Check sheet for the drawn part. Datum: minimum x, y, z corner. Units: mm. Coordinates: 2 decimals unless noted, no trailing zeros. Write each loop counter-clockwise with the first axis right and the second up, starting at its lowest first coordinate (ties: lowest second). Pieces come first, ordered by that corner, then holes. Notation, with made-up numbers: M -26,5.25 L -22,5.25 A25 ccw -22,33.25 Z; hole C 32.25,78.5 d4. An arc over 180 degrees is marked long. Answer as CSV lines item,"result". Start each with the question number.
Q1. Mould release check, pull along Y, two halves, no side actions. Record for the marked faces 1 and 2: pulls with the +Y half, pulls with the -Y half, needs draft (parallel to the pull), parting line crosses it, or undercut.
Q2. Sectioned sample at A-A, the plane x = 49. Record the cut outline in (y, z).
Q3. Sectioned sample at B-B, the plane y = 19. Record the cut outline in (x, z).
Q4. Thickness scan on line 1 along X through (y, z) = (7, 2.8); line 2 along Y through (x, z) = (71.5, 2.65); line 3 along Z through (x, y) = (41, 17). Record the ranges inside material, lowest first. Write a range as from..to.
Q5. Depth check by flat-ended pin: pin 1 Ø0.5 at (x, z) = (81.5, 3.5) entering from -Y; pin 2 Ø5.5 at (x, y) = (44, 9) entering from +Z; pin 3 Ø1.5 at (y, z) = (15.5, 2.5) entering from -X. Enter the tip coordinate at first touch or a pass-through.
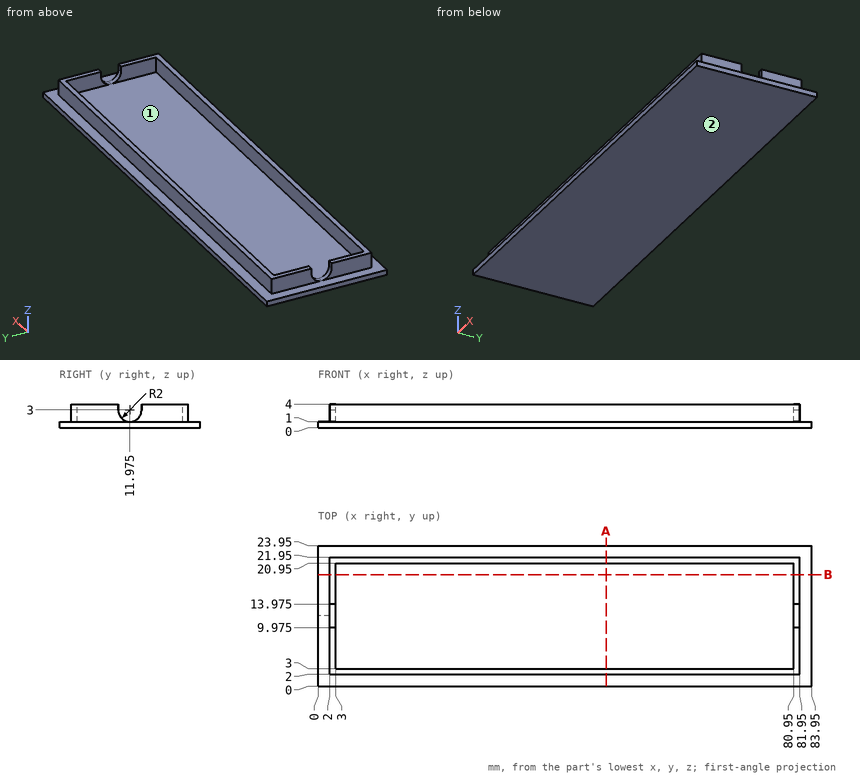
Output:
1,face 1,"undercut"
1,face 2,"needs draft"
2,outline,"M 0,0 L 23.95,0 L 23.95,1 L 21.95,1 L 21.95,4 L 20.95,4 L 20.95,1 L 3,1 L 3,4 L 2,4 L 2,1 L 0,1 Z"
3,outline,"M 0,0 L 83.95,0 L 83.95,1 L 81.95,1 L 81.95,4 L 80.95,4 L 80.95,1 L 3,1 L 3,4 L 2,4 L 2,1 L 0,1 Z"
4,line 1,"x = 2..3, 80.95..81.95"
4,line 2,"y = 2..3, 20.95..21.95"
4,line 3,"z = 0..1"
5,pin 1,"stops at y = 2"
5,pin 2,"stops at z = 1"
5,pin 3,"stops at x = 2"
